The listing builds one solid part. Answer for the finished solid, in the listing's coordinates (mm). A direction names the side the tool comes from. Round coordinates to 2 decimals unless told otherwise and drop trailing zeros. Write each loop counter-clockwise with the first axis right and the second up, starting at its lowest first coordinate (ties: lowest second). Pieces come first, ordered by that corner, then holes.
from build123d import *

# Parameters (mm, degrees)
BOSS_EXTRUDE5_DEPTH      = 25
BOSS_EXTRUDE5_DEPTH_BACK = 1


with BuildPart() as part:
    # Sketch2 → Boss-Extrude5 (new, two sides: drawn at the far end of the back side and taken through both)
    with BuildSketch(Plane.XY.offset(-BOSS_EXTRUDE5_DEPTH_BACK)):
        with BuildLine():
            Line((-32.044117647, 29.926470588), (-32.044117647, 6.926470588))
            Line((-32.044117647, 6.926470588), (-1.044117647, 6.926470588))
            Line((-1.044117647, 6.926470588), (-1.044117647, 29.926470588))
            ThreePointArc((-1.044117647, 29.926470588), (-4.044117647, 32.926470588), (-7.044117647, 29.926470588))
            Line((-7.044117647, 29.926470588), (-7.044117647, 12.926470588))
            Line((-7.044117647, 12.926470588), (-26.044117647, 12.926470588))
            Line((-26.044117647, 12.926470588), (-26.044117647, 29.926470588))
            ThreePointArc((-26.044117647, 29.926470588), (-29.044117647, 32.926470588), (-32.044117647, 29.926470588))
        make_face()
    extrude(amount=BOSS_EXTRUDE5_DEPTH + BOSS_EXTRUDE5_DEPTH_BACK)


solid = part.part
1. Given pin 1 (15 mm diameter, centred on x = -20.5, z = 17, fed in from +Y); pin 2 (4 mm diameter, centred on x = -24, y = 19, fed in from -Z), each flat-ended and moving along its own axis, determine where each tip first touches the part or whether it passes through.
Geometry says:
pin 1: stops at y = 32.74
pin 2: passes through
2. For a pull along X with two mould halves and no side action, classify faces 1 (the face through (-17, 11, -1)), 2 (the face through (-32.044, 19, 12)), 3 (the face through (-1.044, 18, 12)), 4 (the face through (-16, 12.926, 12)) as released by +X, released by -X, zero draft, split by the parting line, or undercut.
Geometry says:
face 1: zero draft
face 2: released by -X
face 3: released by +X
face 4: undercut
3. Section D-D on x = -27.5 is taken. Determine the outline of the cut face in (y, z).
Geometry says:
outline: (6.93, -1) - (32.5, -1) - (32.5, 25) - (6.93, 25) - close
4. Section C-C on x = -14 is taken. Determine the outline of the cut face in (y, z).
Geometry says:
outline: (6.93, -1) - (12.93, -1) - (12.93, 25) - (6.93, 25) - close
5. Straight lines are drawn through the part: line 1 along X through (y, z) = (16.25, 20.25); line 2 along Y through (x, z) = (-14.5, 15.75); line 3 along X through (y, z) = (31.5, 18.5). For each, find the intervals that lie inside material, in ascending order.
Geometry says:
line 1: x = -32.04 to -26.04, -7.04 to -1.04
line 2: y = 6.93 to 12.93
line 3: x = -31.6 to -26.49, -6.6 to -1.49
6. Section B-B on z = 11 is taken. Determine the outline of the cut face in (x, y), plus the area to 3 significant figures.
Geometry says:
outline: (-32.04, 6.93) - (-1.04, 6.93) - (-1.04, 29.93) arc R3 ccw to (-7.04, 29.93) - (-7.04, 12.93) - (-26.04, 12.93) - (-26.04, 29.93) arc R3 ccw to (-32.04, 29.93) - close
area: 418 mm2
7. Section A-A on y = 24.5 is taken. Determine the outline of the cut face in (x, z).
Geometry says:
outline: (-32.04, -1) - (-26.04, -1) - (-26.04, 25) - (-32.04, 25) - close; (-7.04, -1) - (-1.04, -1) - (-1.04, 25) - (-7.04, 25) - close
8. A tool of negligible diameter and unlimited length cuts with its end or side. For faces 5 (the face through (-26.044, 21, 12)), 6 (the face through (-17, 11, 25)), from which of +Z, -Z, +X, -X, +Y, -Y can it reach the whole face along a straight path? Write none if from no direction.
Geometry says:
face 5: +Z, -Z, +Y
face 6: +Z, +X, -X, +Y, -Y
